Read the model definition and answer for the solid it produces. Units are mm, in the model's axes. A direction names the side the tool comes from. Round coordinates to 2 decimals unless told otherwise and drop trailing zeros. Loops run counter-clockwise (first coordinate to the right, second up) from the corner with the lowest first, then second, coordinate; pieces in that order, holes last. Notation, with made-up numbers: M 65.25,-11.5 L 120.25,-11.5 A18 ccw 120.25,15.5 Z; hole C 88,-30.5 d3. An arc over 180 degrees is marked long. Write each question's results on one line, items separated by ' | '.
Autodesk Inventor part; units mm, degrees
ref_plane "Work Plane1" through (0, 10.16, 0) normal (0, 1, 0) x (-1, 0, 0)
ref_plane "YZ Plane" through (0, 0, 0) normal (1, 0, 0) x (0, 1, 0)
ref_plane "XY Plane" through (0, 0, 0) normal (0, 0, 1) x (1, 0, 0)
sketch "Sketch1" plane through (0, 0, 0) normal (0, 1, 0) x (-1, 0, 0)
  circle A0 centre (0, 0) radius 2.3876
  arc A1 (2.9591, 0) -> (1.8161, -2.3362) centre (0, 0) ccw
  line L0 (2.9591, 0) -> (2.3876, 0)
  line L1 (1.8161, -2.3362) -> (1.8161, -17.78)
  line L2 (1.8161, -17.78) -> (2.9591, -17.78)
  line L3 (2.9591, -17.78) -> (2.9591, 0)
  dimension "d0" = 4.7752
  dimension "d1" = 5.9182
  dimension "d2" = 17.78
  dimension "d3" = 1.143
extrude "Extrusion1" add sketch "Sketch1" along normal blind 38.1
ref_plane "Work Plane1" through (0, 10.16, 0) normal (0, 1, 0) x (-1, 0, 0)
sketch "Sketch2" plane through (0, 10.16, 0) normal (0, 1, 0) x (-1, 0, 0)
  circle A0 centre (0, 0) radius 2.3876
  arc A1 (2.9591, 0) -> (1.8161, -2.3362) centre (0, 0) ccw
  line L0 (1.8161, -2.3362) -> (1.8161, -17.78)
  line L1 (1.8161, -17.78) -> (2.9591, -17.78)
  line L2 (2.9591, -17.78) -> (2.9591, 0)
  line L3 (2.9591, 3.4646) -> (-3.1409, 3.4646)
  line L4 (-3.1409, 3.4646) -> (-3.1409, -3.337)
  line L5 (-3.1409, -3.337) -> (2.9591, -3.337)
  line L6 (2.9591, -3.337) -> (2.9591, 3.4646)
  dimension "d7" = 0
  dimension "d8" = 6.1
  dimension "d9" = 21.2446
  dimension "d10" = 14.443
extrude "Extrusion2" cut sketch "Sketch2" along normal blind 17.78 contours L2 L5 L0 A1 | A1 L0 L5 L4 L3 L6
sketch "Sketch3" plane through (-1.8161, 0, -2.3362) normal (1, 0, 0) x (0, 0, -1)
  circle A0 centre (9.0938, 5.08) radius 2.54
  circle A1 centre (9.0938, 33.02) radius 2.54
  line L0 (15.4438, 0) -> (15.4438, 38.1)
  line L1 (0, 0) -> (15.4438, 0)
  line L2 (0, 38.1) -> (15.4438, 38.1)
  point P0 (-2.3362, 0)
  dimension "d13" = 6.35
  dimension "d14" = 5.08
  dimension "d15" = 5.08
  dimension "d17" = 5.08
extrude "Extrusion3" cut sketch "Sketch3" against normal up to next
equation "\"d17\" = d14"
properties part number "Hinge Wall 1"
Item 1: The part is cut by section C-C (x = -0.9). Determine the outline of the cut face in (y, z).
Outcome:
outline: M 0,-2.82 L 10.16,-2.82 L 10.16,-2.21 L 0,-2.21 Z; M 0,2.21 L 10.16,2.21 L 10.16,2.82 L 0,2.82 Z; M 27.94,-2.82 L 38.1,-2.82 L 38.1,-2.21 L 27.94,-2.21 Z; M 27.94,2.21 L 38.1,2.21 L 38.1,2.82 L 27.94,2.82 Z
Item 2: Straight lines are drawn through the part: line 1 (Y direction, x = -2.3, z = -11.43); line 2 (Z direction, x = 0, y = 7.5); line 3 (X direction, y = 24, z = -11.5). For each, find the intervals that lie inside material, in ascending order.
Outcome:
line 1: y = 0 to 2.54, 7.62 to 30.48, 35.56 to 38.1 | line 2: z = -2.96 to -2.39, 2.39 to 2.96 | line 3: x = -2.96 to -1.82
Item 3: The part is cut by section B-B (z = -11.43). Determine the outline of the cut face in (x, y).
Outcome:
outline: M -2.96,0 L -1.82,0 L -1.82,2.54 L -2.96,2.54 Z; M -2.96,7.62 L -1.82,7.62 L -1.82,30.48 L -2.96,30.48 Z; M -2.96,35.56 L -1.82,35.56 L -1.82,38.1 L -2.96,38.1 Z
Item 4: The mould has two halves that part along Y. Classify faces 3 (the face through (-2, 38.1, -7)), 4 (the face through (-2, 0, -7)), 5 (the face through (-2, 27.94, -2)), 6 (the face through (0.52, 32.95, 2.33)): pulls with the +Y half, pulls with the -Y half, needs draft (parallel to the pull), parting line crosses it, or undercut.
Outcome:
face 3: pulls with the +Y half | face 4: pulls with the -Y half | face 5: undercut | face 6: needs draft
Item 5: The part is cut by section A-A (y = 5.08). Determine the outline of the cut face in (x, z).
Outcome:
outline: M -2.96,-17.78 L -1.82,-17.78 L -1.82,-13.97 L -2.96,-13.97 Z; M -2.96,-8.89 L -1.82,-8.89 L -1.82,-2.34 A2.96 ccw long -2.96,0 Z; hole C 0,0 d4.78
Item 6: The part is cut by section D-D (y = 9). Determine the outline of the cut face in (x, z), plus the area to 3 significant figures.
Outcome:
outline: M -2.96,-17.78 L -1.82,-17.78 L -1.82,-2.34 A2.96 ccw long -2.96,0 Z; hole C 0,0 d4.78 | area: 28.1 mm2
Item 7: For faces 1 (the face through (-2.38, 35.54, -11.1)), 2 (the face through (-2, 19, -3.337)), determine the directions among +Z, -Z, +X, -X, +Y, -Y from which every point of the face is accessible in a straight line to the end or side of a thin tool.
Outcome:
face 1: +X, -X | face 2: +Z, +X, -X
Item 8: Flat-ended cylindrical pins translate along their axes: pin 1 (10 mm diameter, centred on y = 22.5, z = -5, fed in from +X); pin 2 (0.9 mm diameter, centred on x = -2.5, y = 17.5, fed in from +Z); pin 3 (2 mm diameter, centred on x = -1, z = -13.5, fed in from -Y); pin 4 (2 mm diameter, centred on x = 1.5, y = 7, fed in from -Z). Find the tip coordinate at first contact, or state that the pin passes through.
Outcome:
pin 1: stops at x = -1.82 | pin 2: stops at z = -3.34 | pin 3: stops at y = 0 | pin 4: stops at z = -2.92
